Design review of the part built by this model. Coordinates are the model's own, in mm. Face numbers are marked on the shaded views. A direction names the side the tool comes from. Round coordinates to 2 decimals unless told otherwise and drop trailing zeros. Write each loop counter-clockwise with the first axis right and the second up, starting at its lowest first coordinate (ties: lowest second). Pieces come first, ordered by that corner, then holes. Notation, with made-up numbers: M -35,68 L 7,68 A20 cw 7,77 Z; hole C -16.75,-3.5 d4. An arc over 180 degrees is marked long. Use CSV: the item, a comma, the result in double quotes.
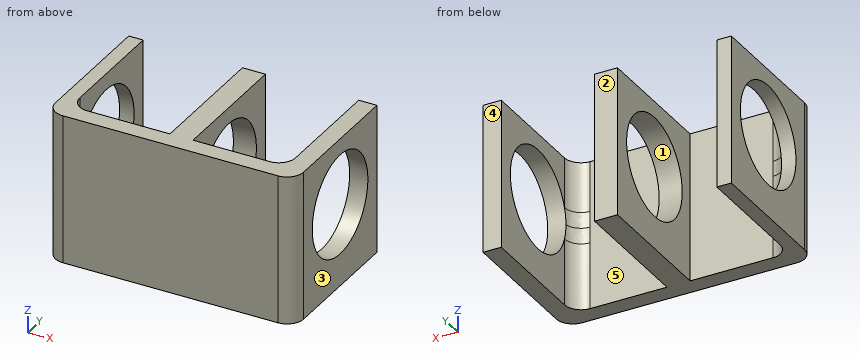
from build123d import *

# Parameters (mm, degrees)
F1_DEPTH = 45
F2_R     = 5
F3_R     = 15.170824
F4_DEPTH = 100
F5_R     = 5


with BuildPart() as f1:
    # F0 (on Top) → F1 (new body)
    with BuildSketch(Plane.XY):
        Polygon((-33.123519, 22.5), (-37.5, 22.5), (-37.5, -22.5), (37.5, -22.5), (37.5, 22.5), (32.003852, 22.5), (32.003852, -17.027041), (3.825535, -17.027041), (3.825535, 22.5), (-3.123519, 22.5), (-3.123519, -17.112833), (-33.123519, -17.112833), align=None)
    extrude(amount=F1_DEPTH)

    # F2
    f2_edges = [f1.edges().sort_by_distance(p)[0] for p in [
        (37.5, -22.5, 22.5),
        (-37.5, -22.5, 22.5),
    ]]
    fillet(f2_edges, radius=F2_R)

    # F3 (on face) → F4 (cut)
    with BuildSketch(Plane(origin=(-37.5, 0, 0), x_dir=(0, -1, 0), z_dir=(-1, 0, 0))):
        with Locations((-2.36058, 24.959255)):
            Circle(F3_R)
    extrude(amount=-F4_DEPTH, mode=Mode.SUBTRACT)

    # F5
    f5_edges = [f1.edges().sort_by_distance(p)[0] for p in [
        (-33.123519, -17.112833, 22.5),
        (32.003852, -17.027041, 22.5),
    ]]
    fillet(f5_edges, radius=F5_R)


solid = f1.part
1) The part is to be moulded in two halves that separate along Y. For the marked faces 1, 2 and 3, say which applies: released by +Y, released by -Y, zero draft, split by the parting line, or undercut.
Answers:
face 1,"undercut"
face 2,"released by +Y"
face 3,"zero draft"
2) Add section A-A on y = 19.5. Write out the cut boundary in (x, z).
Answers:
outline,"M -37.5,0 L -33.12,0 L -33.12,45 L -37.5,45 Z; M -3.12,0 L 3.83,0 L 3.83,45 L -3.12,45 Z; M 32,0 L 37.5,0 L 37.5,45 L 32,45 Z"
3) Machinability: for the marked faces 4 and 5, which of the approach directions +Z, -Z, +X, -X, +Y, -Y give a long, thin tool a straight path to every point of the face, cutting with its end or side? Answer none if there is none.
Answers:
face 4,"+Z, -Z, +X, -X, +Y"
face 5,"+Z, -Z, +Y"
4) For pin 1 Ø5 at (x, y) = (8.5, 10.5) entering from +Z (3 decimals); pin 2 Ø7 at (x, z) = (20, 23) entering from +Y, all flat-tipped, find the tip position at first contact; note any pin that passes through.
Answers:
pin 1,"through"
pin 2,"y = -17.03"
5) Add section D-D on z = 34. Write out the cut boundary in (x, y).
Answers:
outline,"M -37.5,-17.5 A5 ccw -32.5,-22.5 L 32.5,-22.5 A5 ccw 37.5,-17.5 L 37.5,-9.82 L 32,-9.82 L 32,-12.03 A5 cw 27,-17.03 L 3.83,-17.03 L 3.83,-9.82 L -3.12,-9.82 L -3.12,-17.11 L -28.12,-17.11 A5 cw -33.12,-12.11 L -33.12,-9.82 L -37.5,-9.82 Z; M -37.5,14.54 L -33.12,14.54 L -33.12,22.5 L -37.5,22.5 Z; M -3.12,14.54 L 3.83,14.54 L 3.83,22.5 L -3.12,22.5 Z; M 32,14.54 L 37.5,14.54 L 37.5,22.5 L 32,22.5 Z"
6) Add section B-B on z = 41.5. Write out the cut boundary in (x, y), then the cut area to 3 significant figures.
Answers:
outline,"M -37.5,-17.5 A5 ccw -32.5,-22.5 L 32.5,-22.5 A5 ccw 37.5,-17.5 L 37.5,22.5 L 32,22.5 L 32,-12.03 A5 cw 27,-17.03 L 3.83,-17.03 L 3.83,22.5 L -3.12,22.5 L -3.12,-17.11 L -28.12,-17.11 A5 cw -33.12,-12.11 L -33.12,22.5 L -37.5,22.5 Z"
area,"1,070 mm²"
7) Add section C-C on x = -0.5. Write out the cut boundary in (y, z), then the cut area to 3 significant figures.
Answers:
outline,"M -22.5,0 L 22.5,0 L 22.5,45 L -22.5,45 Z; hole C 2.36,24.96 d30.34"
area,"1,300 mm²"
8) Wall thickness on line 1 along X through (y, z) = (18, 3); line 2 along Y through (x, z) = (-11, 31.5); line 3 along Y through (x, z) = (-1, 35.5): over which ranges is each line inside the solid? List them lowest first. Write a range as [from, to].
Answers:
line 1,"[-37.5, -33.12], [-3.12, 3.83], [32, 37.5]"
line 2,"[-22.5, -17.11]"
line 3,"[-22.5, -8.55], [13.27, 22.5]"
